The listing builds one solid part. Answer for the finished solid, in the listing's coordinates (mm). Face numbers are marked on the shaded views. A direction names the side the tool comes from. Give positions to 0.01 mm unless a question says otherwise; leave off trailing zeros. Order: outer loops, then holes, each group sorted by start corner. A loop starts at its lowest first (then second) coordinate and runs counter-clockwise, first axis right, second up. Notation, with made-up numbers: (-30.75, 72.5) - (-22.75, 72.5) arc R20 ccw to (-22.75, 107.5) - close; hole circle Ø5 at (66, 79). An arc over 180 degrees is marked (long way). Answer as a JSON object with one key per item and string values. Group by question number.
Q1. A cutting plane is placed at A-A, the plane y = 45. Give the vertices of the cut face in (x, z).
Q2. The mould has two halves that part along Z. Classify the marked faces 3 and 4: released by +Z, released by -Z, zero draft, split by the parting line, or undercut.
Q3. A cutting plane is placed at C-C, the plane y = 9. Give the vertices of the cut face in (x, z).
Q4. Given pin 1 (2 mm diameter, centred on x = -3, y = -1, fed in from +Z); pin 2 (1 mm diameter, centred on y = 24.5, z = 1.5, fed in from +X); pin 3 (9.5 mm diameter, centred on x = 45.5, y = 0, fed in from +Z); pin 4 (10.5 mm diameter, centred on x = 0, y = 0, fed in from -Z), each flat-ended and moving along its own axis, determine where each tip first touches the part or whether it passes through.
Q5. Consider line 1 (Y direction, x = 0, z = 0.85); line 2 (Y direction, x = 45.5, z = -1.4); line 3 (Z direction, x = 7.5, y = -2). Determine where each line is inside the solid, lowest interval first.
Q6. For the marked faces 1 and 2, determine the directions among +Z, -Z, +X, -X, +Y, -Y from which every point of the face is accessible in a straight line to the end or side of a thin tool.
Q7. A cutting plane is placed at B-B, the plane x = 34. Give the vertices of the cut face in (y, z), and give its area (3 significant figures).
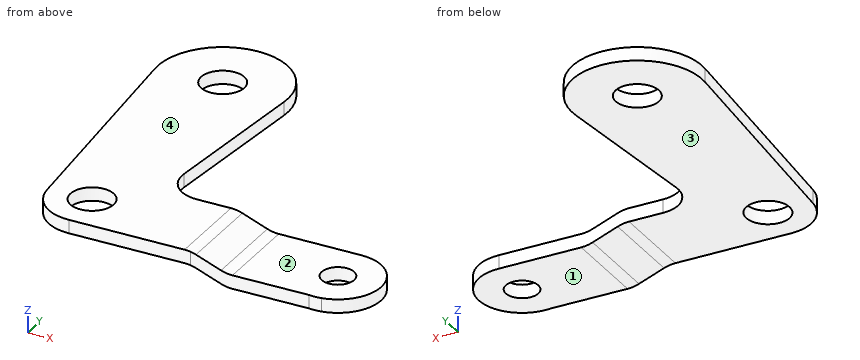
from build123d import *

# Parameters (mm, degrees)
F0_R      = 4
F1_DEPTH  = 2.5
F3_R      = 3
F4_DEPTH  = 2.5
F1_FACE_W = 16
F1_FACE_H = 2.5
F4_FACE_W = 15.976364256
F4_FACE_H = 2.5
F7_R      = 6
F8_R      = 6


with BuildPart() as f1:
    # F0 (on Top) → F1 (new body)
    with BuildSketch(Plane.XY):
        with BuildLine():
            Line((9.1568758371, 14.5686935942), (11.9459763261, 43.8626128117))
            ThreePointArc((11.9459763261, 43.8626128117), (0.0355103222, 56.9999474589), (-11.9524985765, 43.9333333333))
            Line((-11.9524985765, 43.9333333333), (-7.9683323844, -0.7111111111))
            ThreePointArc((-7.9683323844, -0.7111111111), (-5.3995884617, -5.902918299), (0, -8))
            Line((0, -8), (22.5, -8))
            Line((22.5, -8), (22.5, 8))
            Line((22.5, 8), (15.1298640001, 8))
            ThreePointArc((15.1298640001, 8), (10.6907108396, 9.9634272932), (9.1568758371, 14.5686935942))
        make_face()
        Circle(F0_R, mode=Mode.SUBTRACT)
        with Locations((0, 45)):
            Circle(F0_R, mode=Mode.SUBTRACT)
    extrude(amount=-F1_DEPTH)


with BuildPart() as f4:
    # F3 (on offset) → F4 (new body)
    with BuildSketch(Plane(origin=(0, 0, 0), x_dir=(1, 0, 0), z_dir=(0, 0, -1))):
        with BuildLine():
            Line((29.1677432093, -8), (45.5, -8))
            ThreePointArc((45.5, -8), (53.478553963, -0.5853859069), (46.6676332619, 7.914330835))
            Line((46.6676332619, 7.914330835), (44.3885046452, 7.9224098655))
            Line((44.3885046452, 7.9224098655), (29.1677432093, 7.976364256))
            Line((29.1677432093, 7.976364256), (29.1677432093, -8))
        make_face()
        with Locations((45.5, 0)):
            Circle(F3_R, mode=Mode.SUBTRACT)
        with BuildLine():
            Line((44.3885046452, 7.9224098655), (46.6676332619, 7.914330835))
            ThreePointArc((46.6676332619, 7.914330835), (45.5283581353, 7.9999497384), (44.3885046452, 7.9224098655))
        make_face()
    extrude(amount=-F4_DEPTH)


with BuildPart() as f5:
    # F1_face (on face) → F5 section 0
    with BuildSketch(Plane(origin=(22.5, 0, -1.25), x_dir=(0, 1, 0), z_dir=(1, 0, 0))):
        Rectangle(F1_FACE_W, F1_FACE_H)
    # F4_face (on face) → F5 section 1
    with BuildSketch(Plane(origin=(29.1677432093, 0.011817872, 1.25), x_dir=(0, -1, 0), z_dir=(-1, 0, 0))):
        Rectangle(F4_FACE_W, F4_FACE_H)
    loft()


with BuildPart() as f1_1:
    add(f1.part)

    # F6: union F4, F5
    add(f4.part)
    add(f5.part)

    # F7
    f7_edges = [f1_1.edges().sort_by_distance(p)[0] for p in [
        (22.5, 0, 0),
        (29.167743, 0.011818, 2.5),
    ]]
    fillet(f7_edges, radius=F7_R)

    # F8
    f8_edges = [f1_1.edges().sort_by_distance(p)[0] for p in [
        (29.167743, 0.011818, 0),
        (22.5, 0, -2.5),
    ]]
    fillet(f8_edges, radius=F8_R)


with BuildPart() as f9_1:
    # F9: instance of F1
    add(f1_1.part.mirror(Plane.XY))


solid = f9_1.part
Reply:
{
 "1": {"outline": "(-12, 0) - (-4, 0) - (-4, 2.5) - (-12, 2.5) - close; (4, 0) - (12, 0) - (12, 2.5) - (4, 2.5) - close"},
 "2": {"face 3": "released by -Z", "face 4": "released by +Z"},
 "3": {"outline": "(-8.83, 0) - (11.81, 0) - (11.81, 2.5) - (-8.83, 2.5) - close"},
 "4": {"pin 1": "stops at z = 2.5", "pin 2": "stops at x = 10.15", "pin 3": "stops at z = 0", "pin 4": "stops at z = 0"},
 "5": {"line 1": "y = -8 to -4, 4 to 41, 49 to 57", "line 2": "y = -8 to -3, 3 to 8", "line 3": "z = 0 to 2.5"},
 "6": {"face 1": "-Z, +X, -X, +Y, -Y", "face 2": "+Z, +X, +Y, -Y"},
 "7": {"outline": "(-7.96, -2.5) - (8, -2.5) - (8, 0) - (-7.96, 0) - close", "area": "39.9 mm^2"}
}
